Can you work these out from the model? Positions are in its coordinate system, mm. Give positions to 0.01 mm unless a question says otherwise; leave off trailing zeros. Order: outer loops, then holes, each group sorted by start corner. A loop starts at its lowest first (then second) coordinate and runs counter-clockwise, first axis right, second up. Notation, with made-up numbers: M 23,-17.75 L 37,-17.75 A12 ccw 37,-9.75 Z; hole C 20,-36.5 d2. An arc over 180 degrees is marked long. Use a Markdown table: item, result. Add a question column.
from build123d import *

# Parameters (mm, degrees)
F0_R     = 1.5
F1_DEPTH = 1.5


with BuildPart() as f1:
    # F0 (on Top) → F1 (new body)
    with BuildSketch(Plane.XY):
        with BuildLine():
            ThreePointArc((26, 0), (29.183497, 15.104915), (34.266455, 29.680808))
            ThreePointArc((34.266455, 29.680808), (34.47702, 31.713219), (33.516861, 33.516861))
            ThreePointArc((33.516861, 33.516861), (31.713219, 34.47702), (29.680808, 34.266455))
            ThreePointArc((29.680808, 34.266455), (15.104915, 29.183497), (0, 26))
            ThreePointArc((0, 26), (-15.104915, 29.183497), (-29.680808, 34.266455))
            ThreePointArc((-29.680808, 34.266455), (-31.713219, 34.47702), (-33.516861, 33.516861))
            ThreePointArc((-33.516861, 33.516861), (-34.47702, 31.713219), (-34.266455, 29.680808))
            ThreePointArc((-34.266455, 29.680808), (-29.183497, 15.104915), (-26, 0))
            ThreePointArc((-26, 0), (-29.183497, -15.104915), (-34.266455, -29.680808))
            ThreePointArc((-34.266455, -29.680808), (-34.47702, -31.713219), (-33.516861, -33.516861))
            ThreePointArc((-33.516861, -33.516861), (-31.713219, -34.47702), (-29.680808, -34.266455))
            ThreePointArc((-29.680808, -34.266455), (-15.104915, -29.183497), (0, -26))
            ThreePointArc((0, -26), (15.104915, -29.183497), (29.680808, -34.266455))
            ThreePointArc((29.680808, -34.266455), (31.713219, -34.47702), (33.516861, -33.516861))
            ThreePointArc((33.516861, -33.516861), (34.47702, -31.713219), (34.266455, -29.680808))
            ThreePointArc((34.266455, -29.680808), (29.183497, -15.104915), (26, 0))
        make_face()
        with Locations((-29.392136, -29.392136)):
            Circle(F0_R, mode=Mode.SUBTRACT)
        with BuildLine():
            ThreePointArc((-24.324473, -24.324473), (-24.671832, -23.656327), (-24.572337, -22.909884))
            Line((-24.572337, -22.909884), (-21.918806, -17.251149))
            ThreePointArc((-21.918806, -17.251149), (-20.871666, -16.534722), (-19.73736, -17.103157))
            Line((-19.73736, -17.103157), (-18.702974, -18.702974))
            Line((-18.702974, -18.702974), (-17.103157, -19.73736))
            ThreePointArc((-17.103157, -19.73736), (-16.534722, -20.871666), (-17.251149, -21.918806))
            Line((-17.251149, -21.918806), (-22.909884, -24.572337))
            ThreePointArc((-22.909884, -24.572337), (-23.656327, -24.671832), (-24.324473, -24.324473))
        make_face(mode=Mode.SUBTRACT)
        with Locations((-15.25, -15.25)):
            Circle(F0_R, mode=Mode.SUBTRACT)
        with Locations((29.392136, -29.392136)):
            Circle(F0_R, mode=Mode.SUBTRACT)
        with BuildLine():
            Line((21.918806, -17.251149), (24.572337, -22.909884))
            ThreePointArc((24.572337, -22.909884), (24.671832, -23.656327), (24.324473, -24.324473))
            ThreePointArc((24.324473, -24.324473), (23.656327, -24.671832), (22.909884, -24.572337))
            Line((22.909884, -24.572337), (17.251149, -21.918806))
            ThreePointArc((17.251149, -21.918806), (16.534722, -20.871666), (17.103157, -19.73736))
            Line((17.103157, -19.73736), (18.702974, -18.702974))
            Line((18.702974, -18.702974), (19.73736, -17.103157))
            ThreePointArc((19.73736, -17.103157), (20.871666, -16.534722), (21.918806, -17.251149))
        make_face(mode=Mode.SUBTRACT)
        with BuildLine():
            ThreePointArc((8.383883, -15.31353), (8.608023, -16.776019), (7.279787, -17.427863))
            Line((7.279787, -17.427863), (0, -16.125))
            Line((0, -16.125), (-7.279787, -17.427863))
            ThreePointArc((-7.279787, -17.427863), (-8.608023, -16.776019), (-8.383883, -15.31353))
            Line((-8.383883, -15.31353), (-0.883883, -7.81353))
            ThreePointArc((-0.883883, -7.81353), (0, -7.447413), (0.883883, -7.81353))
            Line((0.883883, -7.81353), (8.383883, -15.31353))
        make_face(mode=Mode.SUBTRACT)
        with Locations((15.25, -15.25)):
            Circle(F0_R, mode=Mode.SUBTRACT)
        with BuildLine():
            Line((-16.125, 0), (-17.427863, 7.279787))
            ThreePointArc((-17.427863, 7.279787), (-16.776019, 8.608023), (-15.31353, 8.383883))
            Line((-15.31353, 8.383883), (-7.81353, 0.883883))
            ThreePointArc((-7.81353, 0.883883), (-7.447413, 0), (-7.81353, -0.883883))
            Line((-7.81353, -0.883883), (-15.31353, -8.383883))
            ThreePointArc((-15.31353, -8.383883), (-16.776019, -8.608023), (-17.427863, -7.279787))
            Line((-17.427863, -7.279787), (-16.125, 0))
        make_face(mode=Mode.SUBTRACT)
        with Locations((-15.25, 15.25)):
            Circle(F0_R, mode=Mode.SUBTRACT)
        with BuildLine():
            ThreePointArc((-17.251149, 21.918806), (-16.534722, 20.871666), (-17.103157, 19.73736))
            Line((-17.103157, 19.73736), (-18.702974, 18.702974))
            Line((-18.702974, 18.702974), (-19.73736, 17.103157))
            ThreePointArc((-19.73736, 17.103157), (-20.871666, 16.534722), (-21.918806, 17.251149))
            Line((-21.918806, 17.251149), (-24.572337, 22.909884))
            ThreePointArc((-24.572337, 22.909884), (-24.671832, 23.656327), (-24.324473, 24.324473))
            ThreePointArc((-24.324473, 24.324473), (-23.656327, 24.671832), (-22.909884, 24.572337))
            Line((-22.909884, 24.572337), (-17.251149, 21.918806))
        make_face(mode=Mode.SUBTRACT)
        with Locations((-29.392136, 29.392136)):
            Circle(F0_R, mode=Mode.SUBTRACT)
        with BuildLine():
            ThreePointArc((7.81353, -0.883883), (7.447413, 0), (7.81353, 0.883883))
            Line((7.81353, 0.883883), (15.31353, 8.383883))
            ThreePointArc((15.31353, 8.383883), (16.776019, 8.608023), (17.427863, 7.279787))
            Line((17.427863, 7.279787), (16.125, 0))
            Line((16.125, 0), (17.427863, -7.279787))
            ThreePointArc((17.427863, -7.279787), (16.776019, -8.608023), (15.31353, -8.383883))
            Line((15.31353, -8.383883), (7.81353, -0.883883))
        make_face(mode=Mode.SUBTRACT)
        with BuildLine():
            Line((-7.279787, 17.427863), (0, 16.125))
            Line((0, 16.125), (7.279787, 17.427863))
            ThreePointArc((7.279787, 17.427863), (8.608023, 16.776019), (8.383883, 15.31353))
            Line((8.383883, 15.31353), (0.883883, 7.81353))
            ThreePointArc((0.883883, 7.81353), (0, 7.447413), (-0.883883, 7.81353))
            Line((-0.883883, 7.81353), (-8.383883, 15.31353))
            ThreePointArc((-8.383883, 15.31353), (-8.608023, 16.776019), (-7.279787, 17.427863))
        make_face(mode=Mode.SUBTRACT)
        with Locations((15.25, 15.25)):
            Circle(F0_R, mode=Mode.SUBTRACT)
        with BuildLine():
            Line((19.73736, 17.103157), (18.702974, 18.702974))
            Line((18.702974, 18.702974), (17.103157, 19.73736))
            ThreePointArc((17.103157, 19.73736), (16.534722, 20.871666), (17.251149, 21.918806))
            Line((17.251149, 21.918806), (22.909884, 24.572337))
            ThreePointArc((22.909884, 24.572337), (23.656327, 24.671832), (24.324473, 24.324473))
            ThreePointArc((24.324473, 24.324473), (24.671832, 23.656327), (24.572337, 22.909884))
            Line((24.572337, 22.909884), (21.918806, 17.251149))
            ThreePointArc((21.918806, 17.251149), (20.871666, 16.534722), (19.73736, 17.103157))
        make_face(mode=Mode.SUBTRACT)
        with Locations((29.392136, 29.392136)):
            Circle(F0_R, mode=Mode.SUBTRACT)
    extrude(amount=F1_DEPTH)


solid = f1.part
1. I need wall thicknesses on L1, parallel to Y at x = 5, z = 0.4; L2, parallel to Y at x = 15.25, z = 1.05; L3, parallel to Y at x = -14, z = 1.3. Which ranges of each line are inside material? Lowest first, please. Write a range as [from, to].
2. We'd pull the mould along Y, two halves only. Please class faces 1 (the face through (-15.31, -29.24, 0.74)), 2 (the face through (27.894, -29.326, 0.74)): +Y half, -Y half, draft (parallel to the pull), parting line (faces both ways), or undercut.
3. If we section it at B-B, the plane z = 1: State how many separate pieces and enclosed holes the cut face has, then the cut area to 3 significant figures.
4. If we section it at A-A, the plane x = 4: List the corners of the cut face in (y, z) for me.
Geometry results:
| question | item | result |
|---|---|---|
| 1 | L1 | y = [-26.83, -17.02], [-11.93, 11.93], [17.02, 26.83] |
| 1 | L2 | y = [-29.22, -16.75], [-13.75, -8.32], [8.32, 13.75], [16.75, 29.22] |
| 1 | L3 | y = [-28.88, -16.08], [-14.42, -7.07], [7.07, 14.42], [16.08, 28.88] |
| 2 | face 1 | -Y half |
| 2 | face 2 | undercut |
| 3 | separate pieces | 1 |
| 3 | enclosed holes | 16 |
| 3 | area | 2,960 mm^2 |
| 4 | outline | M -26.65,0 L -16.84,0 L -16.84,1.5 L -26.65,1.5 Z; M -10.93,0 L 10.93,0 L 10.93,1.5 L -10.93,1.5 Z; M 16.84,0 L 26.65,0 L 26.65,1.5 L 16.84,1.5 Z |
